```python
from build123d import *

# Parameters (mm, degrees)
ESQUISSE1_R      = 5
EXTRUSION1_DEPTH = 150
CHANFREIN1_SIZE  = 0.5
ESQUISSE2_R      = 2.5
EXTRUSION2_DEPTH = 15
ESQUISSE3_R      = 2.5
EXTRUSION3_DEPTH = 15


with BuildPart() as part:
    # Esquisse1 → Extrusion1 (new body)
    with BuildSketch(Plane(origin=(0, 0, 0), x_dir=(1, 0, 0), z_dir=(0, 1, 0))):
        Circle(ESQUISSE1_R)
    extrude(amount=EXTRUSION1_DEPTH)

    # Chanfrein1
    chanfrein1_edges = [part.edges().sort_by_distance(p)[0] for p in [
        (-5, 0, 0),
        (-5, 150, 0),
    ]]
    chamfer(chanfrein1_edges, length=CHANFREIN1_SIZE)

    # Esquisse2 → Extrusion2 (cut)
    with BuildSketch(Plane.XZ):
        Circle(ESQUISSE2_R)
    extrude(amount=-EXTRUSION2_DEPTH, mode=Mode.SUBTRACT)

    # Esquisse3 → Extrusion3 (cut)
    with BuildSketch(Plane(origin=(0, 150, 0), x_dir=(1, 0, 0), z_dir=(0, 1, 0))):
        Circle(ESQUISSE3_R)
    extrude(amount=-EXTRUSION3_DEPTH, mode=Mode.SUBTRACT)


solid = part.part
```
Input: part model. Units: mm. Frame: model coordinates. A direction names the side the tool comes from. Coordinates: 2 decimals unless noted, no trailing zeros. Loops run counter-clockwise (first coordinate to the right, second up) from the corner with the lowest first, then second, coordinate; pieces in that order, holes last. Notation, with made-up numbers: M 42.5,14.25 L 47.5,14.25 A36 cw 47.5,48.25 Z; hole C 61,82 d9. An arc over 180 degrees is marked long. Use a Markdown table: item, result. Add a question column.
1) Pin query (flat end, axial travel): P1, Ø5.5, axis at x = 0.5, z = -1, coming from the +Y side; P2, Ø4.5, axis at x = 0, z = 0, coming from the +Y side; P3, Ø2, axis at x = -1.5, y = 61, coming from the -Z side; P4, Ø2.5, axis at x = -1, z = -0.5, coming from the -Y side. Return the tip coordinate at first contact, or that it passes through.
2) Section C-C, the plane y = 84.5. Return the cut outline in (x, z).
3) Line query: L1, parallel to Z at x = 0, y = 139; L2, parallel to Z at x = -0.5, y = 123. Output: solid intervals per line, ascending. Write a range as from..to.
4) Section A-A, the plane x = 0. Return the cut outline in (y, z).
5) Draft query along X for faces 4 (the flat face through (2, 150, 2)), 5 (the flat face through (0, 15, 0)), 6 (the cylindrical face through (-1.08, 73.96, 4.88)). Return one class per face: +X half, -X half, draft (parallel to the pull), parting line (faces both ways), or undercut.
6) Set-up query: faces 1 (the cylindrical face through (-0.54, 142.6, 2.44)), 2 (the cylindrical face through (-0.54, 7.4, -2.44)), 3 (the flat face through (2, 0, 2)). Return all of +Z, -Z, +X, -X, +Y, -Y with unobstructed straight access to the full face (end or side cutting, diameter ignored); none if empty.
7) Section B-B, the plane z = 0. Return the cut outline in (x, y), plus the area to 3 significant figures.
Answer below:
| question | item | result |
|---|---|---|
| 1 | P1 | y = 150 |
| 1 | P2 | y = 135 |
| 1 | P3 | z = -4.97 |
| 1 | P4 | y = 15 |
| 2 | outline | C 0,0 d10 |
| 3 | L1 | -5..-2.5, 2.5..5 |
| 3 | L2 | -4.97..4.97 |
| 4 | outline | M 0,-4.5 L 0.5,-5 L 149.5,-5 L 150,-4.5 L 150,-2.5 L 135,-2.5 L 135,2.5 L 150,2.5 L 150,4.5 L 149.5,5 L 0.5,5 L 0,4.5 L 0,2.5 L 15,2.5 L 15,-2.5 L 0,-2.5 Z |
| 5 | face 4 | draft |
| 5 | face 5 | undercut |
| 5 | face 6 | parting line |
| 6 | face 1 | +Y |
| 6 | face 2 | -Y |
| 6 | face 3 | +Z, -Z, +X, -X, -Y |
| 7 | outline | M -5,0.5 L -4.5,0 L -2.5,0 L -2.5,15 L 2.5,15 L 2.5,0 L 4.5,0 L 5,0.5 L 5,149.5 L 4.5,150 L 2.5,150 L 2.5,135 L -2.5,135 L -2.5,150 L -4.5,150 L -5,149.5 Z |
| 7 | area | 1,350 mm2 |
